from build123d import *

# Parameters (mm, degrees)
F0_R     = 3
F0_R_2   = 14
F1_DEPTH = 60
F2_R     = 7
F3_DEPTH = 25


with BuildPart() as f1:
    # F0 (on Top) → F1 (new body)
    with BuildSketch(Plane.XY):
        Polygon((-52.5, 10), (-52.5, 0), (52.5, 0), (52.5, 10), (27.5, 10), (27.5, 63), (-27.5, 63), (-27.5, 10), align=None)
        with Locations((0, 15)):
            Circle(F0_R, mode=Mode.SUBTRACT)
        with Locations((-19, 34)):
            Circle(F0_R, mode=Mode.SUBTRACT)
        with Locations((0, 34)):
            Circle(F0_R_2, mode=Mode.SUBTRACT)
        with Locations((19, 34)):
            Circle(F0_R, mode=Mode.SUBTRACT)
        with Locations((0, 53)):
            Circle(F0_R, mode=Mode.SUBTRACT)
    extrude(amount=F1_DEPTH)

    # F2 (on face) → F3 (cut)
    with BuildSketch(Plane(origin=(0, 10, 0), x_dir=(-1, 0, 0), z_dir=(0, 1, 0))):
        with Locations((-40, 47)):
            Circle(F2_R)
        with Locations((-40, 12)):
            Circle(F2_R)
        with Locations((40, 47)):
            Circle(F2_R)
        with Locations((40, 12)):
            Circle(F2_R)
    extrude(amount=-F3_DEPTH, mode=Mode.SUBTRACT)


solid = f1.part
Can you work these out from the model? Positions are in its coordinate system, mm. A direction names the side the tool comes from. Give positions to 0.01 mm unless a question says otherwise; leave off trailing zeros. Loops run counter-clockwise (first coordinate to the right, second up) from the corner with the lowest first, then second, coordinate; pieces in that order, holes last. Notation, with made-up numbers: M 17,29 L 70,29 A26 cw 70,53 Z; hole C -14,-27 d7. An arc over 180 degrees is marked long. One line per item, written item: value. Start each with the question number.
1) On a 3-axis mill with a long thin cutter (end or side, diameter ignored), from which of +Z, -Z, +X, -X, +Y, -Y can I reach the whole of each face in a straight line? I mean faces 5 (the face through (-1, 0, 30)), 6 (the face through (-40, 10, 30)), 7 (the face through (27.5, 36, 30)). Say none if no direction works.
2) I'm going to push flat-ended pins straight in: pin 1 (12 mm diameter, centred on y = 43.5, z = 6, fed in from -X); pin 2 (16 mm diameter, centred on x = 40, z = 47, fed in from +Y); pin 3 (5.5 mm diameter, centred on x = 0, y = 15, fed in from +Z); pin 4 (18 mm diameter, centred on x = 40, z = 12, fed in from -Y). Where does each tip first touch, or does it pass through?
3) If we section it at A-A, the plane z = 47: Write out the boundary of the cut face in (x, y).
4) If we section it at D-D, the plane y = 15: Write out the boundary of the cut face in (x, z).
5) If we section it at B-B, the plane y = 34: Write out the boundary of the cut face in (x, z), and give its area (3 significant figures).
6) If we section it at C-C, the plane x = 0: Write out the boundary of the cut face in (y, z).
7) Thinking about a two-plate mould opening in Z: for faces 1 (the face through (-1, 18, 60)), 2 (the face through (40, 10, 30)), 3 (the face through (33.323, 5.07, 49.103)), 4 (the face through (-1, 18, 0)), which applies, +Z half, -Z half, draft (parallel to the pull), parting line (faces both ways), or undercut?
8) If I drill on line 1 (Y direction, x = 0, z = 17.5); line 2 (Y direction, x = 19, z = 45); line 3 (Z direction, x = 42.5, y = 4), over which ranges is the centre line in solid material (lowest first)? Write a range as [from, to].
Completed:
1. face 5: +Z, -Z, +X, -X, -Y
1. face 6: +Z, -Z, -X, +Y
1. face 7: +Z, -Z, +X, +Y
2. pin 1: stops at x = -27.5
2. pin 2: stops at y = 10
2. pin 3: passes through
2. pin 4: stops at y = 0
3. outline: M -52.5,0 L -47,0 L -47,10 L -52.5,10 Z; M -33,0 L 33,0 L 33,10 L 27.5,10 L 27.5,63 L -27.5,63 L -27.5,10 L -33,10 Z; M 47,0 L 52.5,0 L 52.5,10 L 47,10 Z; hole C -19,34 d6; hole C 0,34 d28; hole C 0,15 d6; hole C 0,53 d6; hole C 19,34 d6
4. outline: M -27.5,0 L -3,0 L -3,60 L -27.5,60 Z; M 3,0 L 27.5,0 L 27.5,60 L 3,60 Z
5. outline: M -27.5,0 L -22,0 L -22,60 L -27.5,60 Z; M -16,0 L -14,0 L -14,60 L -16,60 Z; M 14,0 L 16,0 L 16,60 L 14,60 Z; M 22,0 L 27.5,0 L 27.5,60 L 22,60 Z
5. area: 900 mm^2
6. outline: M 0,0 L 12,0 L 12,60 L 0,60 Z; M 18,0 L 20,0 L 20,60 L 18,60 Z; M 48,0 L 50,0 L 50,60 L 48,60 Z; M 56,0 L 63,0 L 63,60 L 56,60 Z
7. face 1: +Z half
7. face 2: draft
7. face 3: undercut
7. face 4: -Z half
8. line 1: y = [0, 12], [18, 20], [48, 50], [56, 63]
8. line 2: y = [0, 31], [37, 63]
8. line 3: z = [0, 5.46], [18.54, 40.46], [53.54, 60]
